```python
from build123d import *

# Parameters (mm, degrees)
F0_R         = 27.5
F1_DEPTH     = 4
F3_DEPTH     = 8
F4_W         = 13
F4_H         = 5
F5_DEPTH     = 25
F6_W         = 10
F6_H         = 3
F7_DEPTH     = 25
F9_DEPTH     = 25
F11_DEPTH    = 25
F13_DEPTH    = 6.5
F15_D        = 2.5
F17_DEPTH    = 25
F18_T1_DEPTH = 11.8336321238
F19_T1_DEPTH = 11.3072792493
F19_T3_DEPTH = 8.9630793076
F21_DEPTH    = 25
F22_R        = 3


# Not quite as in the source:
# - a fillet or chamfer that OpenCascade refuses, or shapes differently, is made with other operations: its cross-section is extruded or revolved along the edge and cut away or added


with BuildPart() as f1:
    # F0 (on Top) → F1 (new body)
    with BuildSketch(Plane.XY):
        Circle(F0_R)
    extrude(amount=F1_DEPTH)

    # F2 (on face) → F3 (join)
    with BuildSketch(Plane.XY.offset(4)):
        with BuildLine():
            ThreePointArc((8.5, 26.1533936612), (4.3030033163, 27.1612621662), (9e-08, 27.5))
            ThreePointArc((9e-08, 27.5), (-4.3030032274, 27.1612621803), (-8.5, 26.1533936612))
            Line((-8.5, 26.1533936612), (-8.5, 22.5))
            Line((-8.5, 22.5), (8.5, 22.5))
            Line((8.5, 22.5), (8.5, 26.1533936612))
        make_face()
    extrude(amount=F3_DEPTH)

    # F4 (on face) → F5 (cut)
    with BuildSketch(Plane.XZ.offset(-22.5)):
        with Locations((0, 6.5)):
            Rectangle(F4_W, F4_H)
    extrude(amount=-F5_DEPTH, mode=Mode.SUBTRACT)

    # F6 (on face) → F7 (cut)
    with BuildSketch(Plane.XZ.offset(-22.5)):
        with Locations((0, 10.5)):
            Rectangle(F6_W, F6_H)
    extrude(amount=-F7_DEPTH, mode=Mode.SUBTRACT)

    # F8 (on face) → F9 (cut)
    with BuildSketch(Plane.XZ.offset(-22.5)):
        Polygon((-5, 12), (-6.5, 9), (-5, 9), align=None)
    extrude(amount=-F9_DEPTH, mode=Mode.SUBTRACT)

    # F10 (on face) → F11 (cut)
    with BuildSketch(Plane.XZ.offset(-22.5)):
        Polygon((5, 9), (6.5, 9), (5, 12), align=None)
    extrude(amount=-F11_DEPTH, mode=Mode.SUBTRACT)

    # F12 (on face) → F13 (join)
    with BuildSketch(Plane.XY.offset(4)):
        with BuildLine():
            Line((3.25, -27.3072792493), (3.25, -21))
            Line((3.25, -21), (-3.25, -21))
            Line((-3.25, -21), (-3.25, -27.3072792493))
            ThreePointArc((-3.25, -27.3072792493), (-1.627854515, -27.4517775322), (0, -27.5))
            ThreePointArc((0, -27.5), (1.627854515, -27.4517775322), (3.25, -27.3072792493))
        make_face()
    extrude(amount=F13_DEPTH)

    # F15 (through all)
    with Locations(Plane(origin=(0, -21, 0), x_dir=(-1, 0, 0), z_dir=(0, 1, 0))):
        with Locations((0, 7.25)):
            Hole(F15_D / 2)

    # F16 (on face) → F17 (cut)
    with BuildSketch(Plane(origin=(0, -21, 0), x_dir=(-1, 0, 0), z_dir=(0, 1, 0))):
        with BuildLine():
            Line((-1.75, 10.5), (-0.25, 8.4747448714))
            ThreePointArc((-0.25, 8.4747448714), (0, 8.5), (0.25, 8.4747448714))
            Line((0.25, 8.4747448714), (1.75, 10.5))
            Line((1.75, 10.5), (-1.75, 10.5))
        make_face()
    extrude(amount=-F17_DEPTH, mode=Mode.SUBTRACT)

    # F18: fillet of radius 1 on 2 edges, made by hand

    # F18_s2 → F18_t1 (cut)
    with BuildSketch(Plane.XZ.offset(18.3326157402)):
        with BuildLine():
            ThreePointArc((0.8850285779, 9.3321414608), (0.6895138592, 8.6947290379), (0.9381231309, 8.0760901835))
            ThreePointArc((0.9381231309, 8.0760901835), (0.6266103523, 8.331600419), (0.25, 8.4747448714))
            Line((0.25, 8.4747448714), (0.8850285779, 9.3321414608))
        make_face()
        with BuildLine():
            ThreePointArc((-0.9381231309, 8.0760901835), (-0.6895138592, 8.6947290379), (-0.8850285779, 9.3321414608))
            Line((-0.8850285779, 9.3321414608), (-0.25, 8.4747448714))
            ThreePointArc((-0.25, 8.4747448714), (-0.6266103523, 8.331600419), (-0.9381231309, 8.0760901835))
        make_face()
    extrude(amount=F18_T1_DEPTH, mode=Mode.SUBTRACT)

    # F19: fillet of radius 1 on 4 edges, made by hand

    # F19_s2 → F19_t1 (cut)
    with BuildSketch(Plane.XZ.offset(18.5)):
        with BuildLine():
            ThreePointArc((3.25, 9.5), (2.9571067812, 10.2071067812), (2.25, 10.5))
            Line((2.25, 10.5), (3.25, 10.5))
            Line((3.25, 10.5), (3.25, 9.5))
        make_face()
        with BuildLine():
            ThreePointArc((-3.25, 9.5), (-2.9571067812, 10.2071067812), (-2.25, 10.5))
            Line((-2.25, 10.5), (-3.25, 10.5))
            Line((-3.25, 10.5), (-3.25, 9.5))
        make_face()
    extrude(amount=F19_T1_DEPTH, mode=Mode.SUBTRACT)

    # F19_s4 → F19_t3 (cut)
    with BuildSketch(Plane.XZ.offset(19.7405911939)):
        with BuildLine():
            ThreePointArc((2.2537635225, 10.5), (1.8038630505, 10.3930787005), (1.4501704647, 10.0951791306))
            Line((1.4501704647, 10.0951791306), (1.75, 10.5))
            Line((1.75, 10.5), (2.2537635225, 10.5))
        make_face()
        with BuildLine():
            ThreePointArc((-1.4501704647, 10.0951791306), (-1.8038630505, 10.3930787005), (-2.2537635225, 10.5))
            Line((-2.2537635225, 10.5), (-1.75, 10.5))
            Line((-1.75, 10.5), (-1.4501704647, 10.0951791306))
        make_face()
    extrude(amount=F19_T3_DEPTH, mode=Mode.SUBTRACT)

    # F20 (on face) → F21 (cut)
    with BuildSketch(Plane(origin=(0, 0, 0), x_dir=(1, 0, 0), z_dir=(0, 0, -1))):
        Polygon((2, -10), (5, -10), (5, 10), (2, 10), (2, 3), (-5, 10), (-9, 10), (1, 0), (-9, -10), (-5, -10), (2, -3), align=None)
    extrude(amount=-F21_DEPTH, mode=Mode.SUBTRACT)

    # F22
    f22_edges = [f1.edges().sort_by_distance(p)[0] for p in [
        (-27.5, 0, 0),
        (-1.5, 6.5, 0),
        (-7, 10, 0),
        (-4, 5, 0),
        (-4, -5, 0),
        (-7, -10, 0),
        (-1.5, -6.5, 0),
        (2, -6.5, 0),
        (3.5, -10, 0),
        (5, 0, 0),
        (3.5, 10, 0),
        (2, 6.5, 0),
    ]]
    fillet(f22_edges, radius=F22_R)


solid = f1.part
```
Check sheet for the modelled part. Datum: model origin and axes. Units: mm. A direction names the side the tool comes from. Round coordinates to 2 decimals unless told otherwise and drop trailing zeros. Order: outer loops, then holes, each group sorted by start corner. A loop starts at its lowest first (then second) coordinate and runs counter-clockwise, first axis right, second up. Notation, with made-up numbers: (38.5, -32) - (82.5, -32) arc R18 ccw to (82.5, -15) - close; hole circle Ø4 at (44.25, 63.25). An arc over 180 degrees is marked (long way). Write item = value, one per line.
Q1. Thickness scan on line 1 along X through (y, z) = (-25.5, 7.25); line 2 along Y through (x, z) = (-2.5, 2.75); line 3 along Z through (x, y) = (0, -24). Record the ranges inside material, lowest first.
Computed:
line_1 = -3.25 to -1.25, 1.25 to 3.25
line_2 = -27.38 to -7.51, -3.49 to 3.49, 7.51 to 27.38
line_3 = 0 to 6
Q2. Go/stop test with flat-tipped pins: pin 1 (4 mm diameter, centred on y = 23.5, z = 9.5, fed in from -X); pin 2 (7 mm diameter, centred on x = 0.5, z = 6, fed in from +Y); pin 3 (0.5 mm diameter, centred on x = -8, z = 3.5, fed in from -Y); pin 4 (12 mm diameter, centred on x = -15.5, y = -2.5, fed in from +Z). Record where each tip stops, or that it passes through.
Computed:
pin_1 = -8.5
pin_2 = 27.5
pin_3 = -26.39
pin_4 = 4
Q3. Tool access check on faces 1 (the face through (-1.597, -7.392, 1.252)), 2 (the face through (-6.5, 25, 6)), 3 (the face through (8.5, 24, 8)). Record the directions out of +Z, -Z, +X, -X, +Y, -Y that give a thin tool (end or side, any length) a straight path to the whole face; none if there is none.
Computed:
face_1 = -Z
face_2 = +Y, -Y
face_3 = +Z, +X, +Y, -Y
Q4. Section check A-A (z = 7.25). Record the boundary of the cut face in (x, y).
Computed:
outline = (-8.5, 22.5) - (-6.5, 22.5) - (-6.5, 26.72) arc R27.5 ccw to (-8.5, 26.15) - close; (-3.25, -27.31) arc R27.5 ccw to (-1.25, -27.47) - (-1.25, -21) - (-3.25, -21) - close; (1.25, -27.47) arc R27.5 ccw to (3.25, -27.31) - (3.25, -21) - (1.25, -21) - close; (6.5, 22.5) - (8.5, 22.5) - (8.5, 26.15) arc R27.5 ccw to (6.5, 26.72) - close
Q5. Draft check along X on faces 4 (the face through (3.25, -24, 7)), 5 (the face through (-3.9, 4.9, 3.5)), 6 (the face through (-8.5, 24, 8)), 7 (the face through (0, -21, 5.8)). Enter one of: pulls with the +X half, pulls with the -X half, needs draft (parallel to the pull), parting line crosses it, or undercut.
Computed:
face_4 = pulls with the +X half
face_5 = undercut
face_6 = pulls with the -X half
face_7 = needs draft
